Could you check a few things on this model? Use its own coordinates, in mm. A direction names the side the tool comes from. Give positions to 0.01 mm unless a question says otherwise; leave off trailing zeros. Write each loop counter-clockwise with the first axis right and the second up, starting at its lowest first coordinate (ties: lowest second). Pieces come first, ordered by that corner, then holes. Notation, with made-up numbers: (30, 6) - (51, 6) arc R37 cw to (51, 44) - close; hole circle Ø3 at (-17, 43.5). An arc over 180 degrees is marked (long way). Answer in a Markdown table with one row per item.
Autodesk Inventor part; units mm, degrees
ref_plane "YZ Plane" through (0, 0, 0) normal (1, 0, 0) x (0, 1, 0)
ref_plane "XZ Plane" through (0, 0, 0) normal (0, 1, 0) x (-1, 0, 0)
ref_plane "XY Plane" through (0, 0, 0) normal (0, 0, 1) x (1, 0, 0)
sketch "Skizze1" plane through (0, 0, 0) normal (0, 0, 1) x (1, 0, 0)
  line L0 (0, -80) -> (0, 80) construction
  line L1 (0, 0) -> (-126.7494, 85.2494) construction
  line L2 (0, 0) -> (174.2009, 85.2494) construction
  circle A0 centre (0, -80) radius 10
  line L3 (9.9263, -81.2121) -> (18.5, -11)
  line L4 (-9.9263, -81.2121) -> (-18.5, -11)
  arc A1 (11.1647, -27.3337) -> (6.298, -22.158) centre (7.3916, -26.0056) ccw
  arc A2 (-6.298, -22.158) -> (6.298, -22.158) centre (0, 0) ccw
  arc A3 (-6.298, -22.158) -> (-11.3621, -26.4905) centre (-7.3916, -26.0056) ccw
  circle A4 centre (0, 0) radius 10
  circle A5 centre (0, 0) radius 80 construction
  circle A6 centre (-66.3822, 44.6475) radius 10
  line L5 (-71.4336, 36.0171) -> (-18.5, -11)
  line L6 (-60.2936, 52.5803) -> (0, 21.0429)
  circle A7 centre (71.857, 35.1649) radius 10
  line L7 (18.5, -11) -> (75.6826, 25.9257)
  line L8 (0, 21.0429) -> (66.9086, 43.8548)
  line L9 (-11.3621, -26.4905) -> (-6.9853, -62.3337)
  arc A8 (-6.9853, -62.3337) -> (-4.1667, -63.9094) centre (-5, -62.0913) ccw
  arc A9 (4.1667, -63.9094) -> (-4.1667, -63.9094) centre (0, -73) ccw
  arc A10 (4.1667, -63.9094) -> (6.9853, -62.3337) centre (5, -62.0913) ccw
  line L10 (6.9853, -62.3337) -> (11.1647, -27.3337)
  dimension "d4" = 80
  dimension "d7" = 120
  dimension "d8" = 20
  dimension "d10" = 11
  dimension "d11" = 11
  dimension "d12" = 20
  dimension "d17" = 4
  dimension "d21" = 160
  dimension "d31" = 37
  dimension "d32" = 37
  dimension "d35" = 14
  dimension "d39" = 2
  dimension "d40" = 35.8432
  dimension "d41" = 7
  dimension "d43" = 35
  dimension "d71" = 10
  dimension "d77" = 10
extrude "Extrusion2" add sketch "Skizze1" along normal blind 10 contours A0 | A0 L4 L5 A6 L6 L8 A7 L7 L3 | A6 | A7 | L10 A10 A9 A8 L9 A3 A2 A1
sketch "Skizze4" plane through (0, 0, 10) normal (0, 0, 1) x (1, 0, 0)
  arc A0 (-9.9263, -81.2121) -> (9.9263, -81.2121) centre (0, -80) ccw
  point P0 (0, 0)
hole "Bohrung1" at (0, -80, 10) direction (0, 0, -1) diameter 10 depth 10
sketch "Skizze5" plane through (0, 0, 10) normal (0, 0, 1) x (1, 0, 0)
  arc A0 (-60.2936, 52.5803) -> (-71.4336, 36.0171) centre (-66.3822, 44.6475) ccw
  arc A1 (75.6826, 25.9257) -> (66.9086, 43.8548) centre (71.857, 35.1649) ccw
  point P0 (0, 0)
hole "Bohrung2" at (-66.3822, 44.6475, 10) at (71.857, 35.1649, 10) direction (0, 0, -1) diameter 10 depth 10
fillet "Rundung1" radius 30 3 edges at (0, 21.0429, 5) (18.5, -11, 5) (-18.5, -11, 5)
sketch "Skizze6" plane through (0, 0, 10) normal (0, 0, 1) x (1, 0, 0)
  circle A0 centre (-66.3822, 44.6475) radius 5
  line L0 (0, 0) -> (-66.3822, 44.6475) construction
  arc A1 (-12.9165, 17.7381) -> (-21.4837, 4.4641) centre (0, 0) ccw
  circle A2 centre (0, 0) radius 10
  arc A3 (-12.9165, 17.7381) -> (-13.2992, 22.9189) centre (-14.7162, 20.2097) ccw
  line L1 (-13.2992, 22.9189) -> (-43.9218, 38.9365)
  arc A4 (-43.9218, 38.9365) -> (-47.8486, 37.4608) centre (-45.2257, 36.4437) ccw
  arc A5 (-52.7377, 30.1917) -> (-47.8486, 37.4608) centre (-66.3822, 44.6475) ccw
  arc A6 (-52.7377, 30.1917) -> (-52.6749, 26.0427) centre (-50.8067, 28.1459) ccw
  line L2 (-52.6749, 26.0427) -> (-26.5076, 2.8001)
  arc A7 (-26.5076, 2.8001) -> (-21.4837, 4.4641) centre (-24.4772, 5.0861) ccw
  line L3 (-71.4336, 36.0171) -> (-26.9812, -3.4668)
  line L4 (-11.4042, 27.008) -> (-60.2936, 52.5803)
  dimension "d61" = 10
  dimension "d62" = 5
  dimension "d63" = 5
  dimension "d64" = 18
  dimension "d66" = 25
  dimension "d67" = 35
  dimension "d68" = 5
extrude "Extrusion4" cut sketch "Skizze6" against normal blind 10 contours A1 A7 L2 A6 A5 A4 L1 A3
pattern_circular "Runde Anordnung1" count 2 over 120 about axis through (0, 0, 0) along (0, 0, -1) of "Extrusion4"
extrude "Extrusion5" cut sketch "Skizze1" along normal blind 10 contours L10 A10 A9 A8 L9 A3 A2 A1
equation "\"d32\" = d31"
equation "\"d62\" = 0.5 * d61"
equation "\"d63\" = 0.5 * d61"
properties part number "yoyo" material "Stahl, galvanisiert"
1) Will these pins go through, and if not, where does the flat tip stop? P1, Ø3, axis at y = 5, z = 3, coming from the +X side; P2, Ø1.5, axis at x = 57.5, z = 1.5, coming from the +Y side; P3, Ø2, axis at y = -38, z = 8, coming from the -X side.
Check values:
| item | result |
|---|---|
| P1 | stops at x = 45.6 |
| P2 | stops at y = 40.9 |
| P3 | stops at x = -15.33 |
2) Imagine slicing it at C-C (y = 14). List the corners of the cut face in (x, z) for me, then the cut area to 3 significant figures.
Check values:
| item | result |
|---|---|
| outline | (-46.65, 0) - (-39.12, 0) - (-39.12, 10) - (-46.65, 10) - close; (-16.9, 0) - (16.9, 0) - (16.9, 10) - (-16.9, 10) - close; (48.48, 0) - (57.21, 0) - (57.21, 10) - (48.48, 10) - close |
| area | 501 mm2 |
3) Imagine slicing it at D-D (x = -55.5). List the corners of the cut face in (y, z) for me.
Check values:
| item | result |
|---|---|
| outline | (21.86, 0) - (50.07, 0) - (50.07, 10) - (21.86, 10) - close |
4) If I drill on line 1 (Y direction, x = -5.5, z = 2.5); line 2 (X direction, y = 5, z = 7.25); line 3 (X direction, y = -49, z = 8.25), over which ranges is the centre line in solid material (lowest first)?
Check values:
| item | result |
|---|---|
| line 1 | y = -88.35 to -64.03, -22.37 to -8.35, 8.35 to 24.68 |
| line 2 | x = -36.51 to -28.98, -21.37 to -8.66, 8.66 to 21.37, 34.29 to 43.28 |
| line 3 | x = -13.86 to -8.61, 8.58 to 13.86 |
5) Imagine slicing it at B-B (x = 0). List the corners of the cut face in (y, z) for me, then the cut area to 3 significant figures.
Check values:
| item | result |
|---|---|
| outline | (-90, 0) - (-85, 0) - (-85, 10) - (-90, 10) - close; (-75, 0) - (-63, 0) - (-63, 10) - (-75, 10) - close; (-23.04, 0) - (-10, 0) - (-10, 10) - (-23.04, 10) - close; (10, 0) - (23.7, 0) - (23.7, 10) - (10, 10) - close |
| area | 437 mm2 |
6) Imagine slicing it at A-A (y = -35). List the corners of the cut face in (x, z) for me.
Check values:
| item | result |
|---|---|
| outline | (-15.57, 0) - (-10.32, 0) - (-10.32, 10) - (-15.57, 10) - close; (10.25, 0) - (15.57, 0) - (15.57, 10) - (10.25, 10) - close |
7) On a 3-axis mill with a long thin cutter (end or side, diameter ignored), from which of +Z, -Z, +X, -X, +Y, -Y can I reach the whole of each face in a straight line? I mean faces 4 (the face through (32.517, 27.154, 5.07)), 5 (the face through (0.033, 23.693, 5.07)). Say none if no direction works.
Check values:
| item | result |
|---|---|
| face 4 | +Z, -Z |
| face 5 | +Z, -Z, +Y |
8) We'd pull the mould along X, two halves only. Please class faces 1 (the face through (52.674, 11.068, 4.93)), 2 (the face through (0, -63, 5)), 3 (the face through (2, -12, 10)): +X half, -X half, draft (parallel to the pull), parting line (faces both ways), or undercut.
Check values:
| item | result |
|---|---|
| face 1 | +X half |
| face 2 | undercut |
| face 3 | draft |
